Input: part model. Units: mm. Frame: model coordinates. Face numbers are marked on the shaded views. Coordinates: 2 decimals unless noted, no trailing zeros. Write each loop counter-clockwise with the first axis right and the second up, starting at its lowest first coordinate (ties: lowest second). Pieces come first, ordered by that corner, then holes. Notation, with made-up numbers: (-21, 86.25) -> (-7, 86.25) arc R31 cw to (-7, 111.25) -> close; hole circle Ø6 at (61, -32). An arc over 180 degrees is marked (long way). Use one line per item in the form item = value. Start each with the question number.
(1) Ray query, line 1 along X through (y, z) = (-4, -0.9); line 2 along Y through (x, z) = (-22, -0.8); line 3 along X through (y, z) = (1.5, -0.3). Return the intervals inside material, ascending.
(2) Cut plane B-B on y = 0. Return the cut outline in (x, z), plus the area to 4 significant figures.
(3) Cut plane A-A on x = 20. Return the cut outline in (y, z), plus the area to 4 significant figures.
(4) First-contact query: pin 1 (4.5 mm diameter, centred on x = 20, y = 0, fed in from -Z); pin 2 (12 mm diameter, centred on x = -22, y = 3, fed in from +Z); pin 3 (2 mm diameter, centred on x = -35, y = 3.5, fed in from +Z). Flat tips, straight axial feed; report the tip coordinate or a pass-through.
(5) Cut plane D-D on y = 6. Return the cut outline in (x, z).
(6) Cut plane C-C on x = -26.5. Return the cut outline in (y, z), plus the area to 4 significant figures.
(7) Pull-direction query (Y, two-part tool) for the marked faces 1 and 2; classes: released by +Y, released by -Y, zero draft, split by the parting line, or undercut.
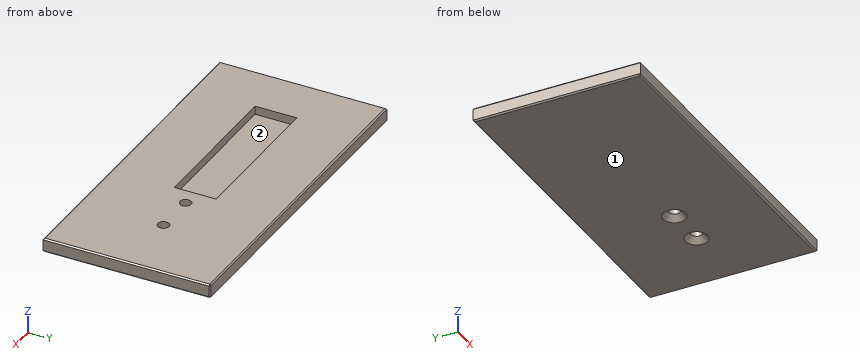
Autodesk Inventor part; units mm, degrees
ref_plane "YZ Plane" through (0, 0, 0) normal (1, 0, 0) x (0, 1, 0)
ref_plane "XZ Plane" through (0, 0, 0) normal (0, 1, 0) x (-1, 0, 0)
ref_plane "XY Plane" through (0, 0, 0) normal (0, 0, 1) x (1, 0, 0)
sketch "Szkic1" plane through (0, 0, 0) normal (0, 0, 1) x (1, 0, 0)
  line L0 (-60, -30) -> (60, -30)
  line L1 (60, -30) -> (60, 30)
  line L2 (60, 30) -> (-60, 30)
  line L3 (-60, 30) -> (-60, -30)
  line L4 (-60, -30) -> (60, 30) construction
  line L5 (60, -30) -> (-60, 30) construction
  point P0 (0, 0)
  dimension "d0" = 120
  dimension "d1" = 60
extrude "Wyciągnięcie proste1" add sketch "Szkic1" against normal blind 5
sketch "Szkic2" plane through (0, 0, 0) normal (0, 0, 1) x (1, 0, 0)
  circle A0 centre (-35, 0) radius 2.5
  circle A1 centre (-20, 0) radius 2.5
  circle A2 centre (20, 0) radius 2
  circle A3 centre (35, 0) radius 2
  line L0 (-39.7, -6.05) -> (-39.7, 6.05)
  line L1 (39.7, -6.05) -> (-39.7, -6.05)
  line L2 (39.7, 6.05) -> (39.7, -6.05)
  line L3 (-39.7, 6.05) -> (39.7, 6.05)
  line L4 (-41.5, 7.5) -> (13.5, 7.5)
  line L5 (13.5, 7.5) -> (13.5, -7.5)
  line L6 (13.5, -7.5) -> (-41.5, -7.5)
  line L7 (-41.5, -7.5) -> (-41.5, 7.5)
  line L8 (-41.5, 7.5) -> (13.5, -7.5) construction
  line L9 (13.5, 7.5) -> (-41.5, -7.5) construction
  point P0 (0, 0)
  point P1 (-14, 0)
  dimension "d4" = 55
  dimension "d5" = 15
  dimension "d6" = 14
extrude "Wyciągnięcie proste2" cut sketch "Szkic2" against normal blind 3 contours A0 | A1 | L1 L5 L6 L7 L4 L3 L0 | L0 L3 L5 L1
sketch "Szkic3" plane through (0, 0, 0) normal (0, 0, 1) x (1, 0, 0)
  circle A0 centre (35, 0) radius 2
  circle A1 centre (20, 0) radius 2
  point P0 (0, 0)
extrude "Wyciągnięcie proste3" cut sketch "Szkic3" against normal through all
thread "Gwint1"
thread "Gwint2"
chamfer "Faza2" distance 0.5 angle 45 9 edges at (60, 30, -2.5) (0, 30, 0) (0, 30, -5) (60, 0, 0) (60, 0, -5) (0, -30, 0) (0, -30, -5) (-60, 0, 0) (-60, 0, -5)
chamfer "Faza3" distance 2 angle 45 2 edges at (18, 0, -5) (33, 0, -5)
properties part number "podstwa" material "MDF — płyta pilśniowa o średniej gęstości"
Values:
q1.line_1 = -60 to -41.5, 13.5 to 60
q1.line_2 = -30 to -7.5, 7.5 to 30
q1.line_3 = -59.8 to -41.5, 13.5 to 18.68, 21.32 to 33.68, 36.32 to 59.8
q2.outline = (-60, -4.5) -> (-59.5, -5) -> (16, -5) -> (18, -3) -> (18, 0) -> (13.5, 0) -> (13.5, -3) -> (-41.5, -3) -> (-41.5, 0) -> (-59.5, 0) -> (-60, -0.5) -> close; (22, -3) -> (24, -5) -> (31, -5) -> (33, -3) -> (33, 0) -> (22, 0) -> close; (37, -3) -> (39, -5) -> (59.5, -5) -> (60, -4.5) -> (60, -0.5) -> (59.5, 0) -> (37, 0) -> close
q2.area = 386.5 mm2
q3.outline = (-30, -4.5) -> (-29.5, -5) -> (-4, -5) -> (-2, -3) -> (-2, 0) -> (-29.5, 0) -> (-30, -0.5) -> close; (2, -3) -> (4, -5) -> (29.5, -5) -> (30, -4.5) -> (30, -0.5) -> (29.5, 0) -> (2, 0) -> close
q3.area = 275.5 mm2
q4.pin_1 = -3.25
q4.pin_2 = 0
q4.pin_3 = -3
q5.outline = (-60, -4.5) -> (-59.5, -5) -> (59.5, -5) -> (60, -4.5) -> (60, -0.5) -> (59.5, 0) -> (13.5, 0) -> (13.5, -3) -> (-41.5, -3) -> (-41.5, 0) -> (-59.5, 0) -> (-60, -0.5) -> close
q6.outline = (-30, -4.5) -> (-29.5, -5) -> (29.5, -5) -> (30, -4.5) -> (30, -0.5) -> (29.5, 0) -> (7.5, 0) -> (7.5, -3) -> (-7.5, -3) -> (-7.5, 0) -> (-29.5, 0) -> (-30, -0.5) -> close
q6.area = 254.5 mm2
q7.face_1 = zero draft
q7.face_2 = undercut
